Verification items for the finished model (mm, model axes). Face numbers are marked on the shaded views. A direction names the side the tool comes from. Give positions to 0.01 mm unless a question says otherwise; leave off trailing zeros. Order: outer loops, then holes, each group sorted by start corner. A loop starts at its lowest first (then second) coordinate and runs counter-clockwise, first axis right, second up.
from build123d import *

# Parameters (mm, degrees)
SKETCH_1_R          = 1.45
EXTRUDE_1_DEPTH     = 25
SKETCH_2_R          = 2.65
EXTRUDE_2_DEPTH     = 1.7
CUT_EXTRUDE_START   = -1
SKETCH_3_W          = 1
SKETCH_3_H          = 1
CUT_EXTRUDE_1_DEPTH = 1
FILLET_1_R          = 0.5
FILLET_2_R          = 1
FILLET_3_R          = 0.5


with BuildPart() as part:
    # 草图1 → 凸台-拉伸1 (new body)
    with BuildSketch(Plane(origin=(0, 0, 0), x_dir=(1, 0, 0), z_dir=(0, 1, 0))):
        with Locations(Location((0, 0, 0), (0, 0, 270))):
            Circle(SKETCH_1_R)
    extrude(amount=EXTRUDE_1_DEPTH)

    # 草图2 → 凸台-拉伸2 (add)
    with BuildSketch(Plane(origin=(0, 25, 0), x_dir=(1, 0, 0), z_dir=(0, 1, 0))):
        with Locations(Location((0, 0, 0), (0, 0, 270))):
            Circle(SKETCH_2_R)
    extrude(amount=EXTRUDE_2_DEPTH)

    # 草图3 → 切除-拉伸1 (cut)
    with BuildSketch(Plane(origin=(0, 26.7, 0), x_dir=(1, 0, 0), z_dir=(0, 1, 0)).offset(CUT_EXTRUDE_START)):
        with BuildLine():
            Line((-0.5, 0.5), (-2.602402736, 0.5))
            ThreePointArc((-2.602402736, 0.5), (-2.65, 0), (-2.602402736, -0.5))
            Line((-2.602402736, -0.5), (-0.5, -0.5))
            Line((-0.5, -0.5), (-0.5, 0.5))
        make_face()
        with Locations((0, 1)):
            Rectangle(SKETCH_3_W, SKETCH_3_H)
        Rectangle(SKETCH_3_W, SKETCH_3_H)
        with Locations((0, -1)):
            Rectangle(SKETCH_3_W, SKETCH_3_H)
        with BuildLine():
            ThreePointArc((2.65, 0), (2.638073848, 0.251130195), (2.602402736, 0.5))
            Line((2.602402736, 0.5), (0.5, 0.5))
            Line((0.5, 0.5), (0.5, -0.5))
            Line((0.5, -0.5), (2.602402736, -0.5))
            ThreePointArc((2.602402736, -0.5), (2.638073848, -0.251130195), (2.65, 0))
        make_face()
    extrude(amount=CUT_EXTRUDE_1_DEPTH, mode=Mode.SUBTRACT)

    # 圆角1
    fillet_1_edges = [part.edges().sort_by_distance(p)[0] for p in [
        (-0.5, 26.2, 0.5),
        (-0.5, 26.2, -0.5),
        (0.5, 26.2, -0.5),
        (0.5, 26.2, 0.5),
    ]]
    fillet(fillet_1_edges, radius=FILLET_1_R)

    # 圆角2
    fillet_2_edges = [part.edges().sort_by_distance(p)[0] for p in [
        (0, 26.7, -2.65),
        (1.687824043, 26.7, 2.042975771),
    ]]
    fillet(fillet_2_edges, radius=FILLET_2_R)

    # 圆角3
    fillet_3_edges = [part.edges().sort_by_distance(p)[0] for p in [
        (0, 25, -2.65),
    ]]
    fillet(fillet_3_edges, radius=FILLET_3_R)


solid = part.part
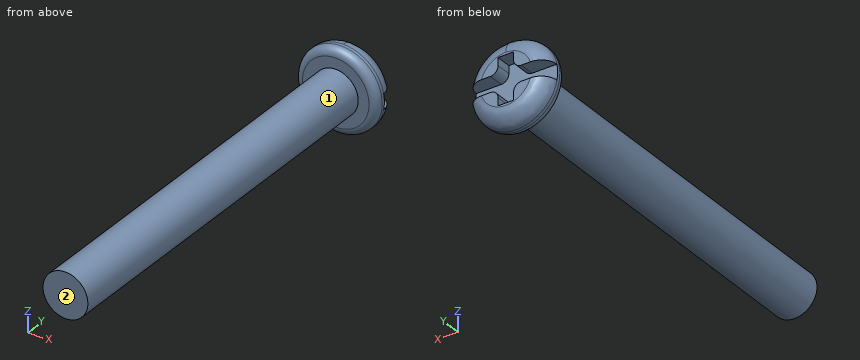
(1) Go/stop test with flat-tipped pins: pin 1 (0.9 mm diameter, centred on x = 0, z = 0, fed in from +Y); pin 2 (3 mm diameter, centred on y = 3, z = 1, fed in from -X); pin 3 (0.8 mm diameter, centred on x = 2, y = 26.5, fed in from -Z). Record where each tip stops, or that it passes through.
Solved:
pin 1: stops at y = 25.7
pin 2: stops at x = -1.45
pin 3: stops at z = -1.83
(2) Section check A-A, the plane z = 0. Enter the section's corners in (x, y), then the cut area to 3 significant figures.
Solved:
outline: (-2.65, 25.5) arc R0.5 ccw to (-2.15, 25) - (-1.45, 25) - (-1.45, 0) - (1.45, 0) - (1.45, 25) - (2.15, 25) arc R0.5 ccw to (2.65, 25.5) - (2.65, 25.7) - (-2.65, 25.7) - close
area: 76.1 mm2
(3) Scan lines: line 1 (Z direction, x = 0.1, y = 20.5); line 2 (Y direction, x = -1.1, z = -0.1); line 3 (X direction, y = 18, z = 1). Record each from-to range of solid material in increasing order.
Solved:
line 1: z = -1.45 to 1.45
line 2: y = 0 to 25.7
line 3: x = -1.05 to 1.05
(4) Set-up check for the marked faces 1 and 2: record each of +Z, -Z, +X, -X, +Y, -Y from which the full face is reachable in a straight line by a thin tool's end or side.
Solved:
face 1: -Y
face 2: +Z, -Z, +X, -X, -Y
(5) Section check B-B, the plane y = 11.75. Enter the section's corners in (x, z), then the cut area to 3 significant figures.
Solved:
outline: circle Ø2.9 at (0, 0)
area: 6.61 mm2
